Geometry check sheet. Reference: the model listing, model coordinates, mm. A direction names the side the tool comes from. Coordinates: 2 decimals unless noted, no trailing zeros. Write each loop counter-clockwise with the first axis right and the second up, starting at its lowest first coordinate (ties: lowest second). Pieces come first, ordered by that corner, then holes. Notation, with made-up numbers: M 42,21 L 47,21 A25 cw 47,60 Z; hole C 50.25,19 d9. An arc over 180 degrees is marked long. Write each question's results on one line, items separated by ' | '.
```python
from build123d import *

# Parameters (mm, degrees)
SKETCH_1_W          = 15.8
SKETCH_1_H          = 15.600000042
EXTRUDE_2_DEPTH     = 6.4
CUT_EXTRUDE_1_DEPTH = 3.2
SKETCH_3_R          = 2.400000003
EXTRUDE_3_DEPTH     = 1.7
SKETCH_4_R          = 2.4
EXTRUDE_4_DEPTH     = 1.7
CUT_EXTRUDE_2_DEPTH = 1.8
SKETCH_6_R          = 2.5
CUT_EXTRUDE_3_DEPTH = 1.8


with BuildPart() as part:
    # Эскиз1 → Бобышка-Вытянуть2 (new body)
    with BuildSketch(Plane(origin=(0, 0, 0), x_dir=(1, 0, 0), z_dir=(0, 1, 0))):
        Rectangle(SKETCH_1_W, SKETCH_1_H)
    extrude(amount=EXTRUDE_2_DEPTH)

    # Эскиз2 → Вырез-Вытянуть1 (cut)
    with BuildSketch(Plane(origin=(0, 6.4, 0), x_dir=(1, 0, 0), z_dir=(0, 1, 0))):
        Polygon((7.9, 0), (0, 0), (-7.9, 0), (-7.9, -7.800000021), (7.9, -7.800000021), align=None)
    extrude(amount=-CUT_EXTRUDE_1_DEPTH, mode=Mode.SUBTRACT)

    # Эскиз3 → Бобышка-Вытянуть3 (add)
    with BuildSketch(Plane(origin=(0, 3.2, 0), x_dir=(1, 0, 0), z_dir=(0, 1, 0))):
        with Locations(Location((-4, -3.900000021, 0), (0, 0, 270))):
            Circle(SKETCH_3_R)
        with Locations(Location((3.874, -3.900000021, 0), (0, 0, 270))):
            Circle(SKETCH_3_R)
    extrude(amount=EXTRUDE_3_DEPTH)

    # Эскиз4 → Бобышка-Вытянуть4 (add)
    with BuildSketch(Plane(origin=(0, 6.4, 0), x_dir=(1, 0, 0), z_dir=(0, 1, 0))):
        with Locations(Location((-4, 3.900000021, 0), (0, 0, 270))):
            Circle(SKETCH_4_R)
        with Locations(Location((3.874, 3.900000021, 0), (0, 0, 270))):
            Circle(SKETCH_4_R)
    extrude(amount=EXTRUDE_4_DEPTH)

    # Эскиз5 → Вырез-Вытянуть2 (cut)
    with BuildSketch(Plane.XZ):
        with BuildLine():
            ThreePointArc((2.241714395, 5.006669145), (0, 6.400000011), (-2.241714395, 5.006669145))
            Line((-2.241714395, 5.006669145), (0, 3.900000011))
            Line((0, 3.900000011), (2.241714395, 5.006669145))
        make_face()
        with BuildLine():
            Line((0, 3.900000011), (-2.241714395, 5.006669145))
            ThreePointArc((-2.241714395, 5.006669145), (-2.5, 3.900000011), (-2.241714395, 2.793330876))
            Line((-2.241714395, 2.793330876), (0, 3.900000011))
        make_face()
        with BuildLine():
            Line((0, 3.900000011), (-2.241714395, 2.793330876))
            ThreePointArc((-2.241714395, 2.793330876), (0, 1.400000011), (2.241714395, 2.793330876))
            Line((2.241714395, 2.793330876), (0, 3.900000011))
        make_face()
        with BuildLine():
            Line((2.241714395, 5.006669145), (0, 3.900000011))
            Line((0, 3.900000011), (2.241714395, 2.793330876))
            ThreePointArc((2.241714395, 2.793330876), (2.434572446, 3.331794936), (2.5, 3.900000011))
            ThreePointArc((2.5, 3.900000011), (2.434572446, 4.468205085), (2.241714395, 5.006669145))
        make_face()
    extrude(amount=-CUT_EXTRUDE_2_DEPTH, mode=Mode.SUBTRACT)

    # Эскиз6 → Вырез-Вытянуть3 (cut)
    with BuildSketch(Plane.XZ):
        with Locations(Location((0, -3.934549789, 0), (0, 0, 270))):
            Circle(SKETCH_6_R)
    extrude(amount=-CUT_EXTRUDE_3_DEPTH, mode=Mode.SUBTRACT)


solid = part.part
```
Q1. Sectioned sample at C-C on z = -3.75. Record the cut outline in (x, y).
Geometry check:
outline: M -7.9,0 L -2.49,0 L -2.49,1.8 L 2.49,1.8 L 2.49,0 L 7.9,0 L 7.9,6.4 L 6.27,6.4 L 6.27,8.1 L 1.48,8.1 L 1.48,6.4 L -1.6,6.4 L -1.6,8.1 L -6.4,8.1 L -6.4,6.4 L -7.9,6.4 Z
Q2. Mould release check, pull along X, two halves, no side actions. Record for faces 1 (the flat face through (-7.9, 2, -2)), 2 (the flat face through (0, 3, -7.8)), 3 (the flat face through (0, 3.2, 4)): pulls with the +X half, pulls with the -X half, needs draft (parallel to the pull), parting line crosses it, or undercut.
Geometry check:
face 1: pulls with the -X half | face 2: needs draft | face 3: undercut
Q3. Sectioned sample at B-B on x = 0. Record the cut outline in (y, z), and give its area (3 significant figures).
Geometry check:
outline: M 0,-7.8 L 6.4,-7.8 L 6.4,0 L 3.2,0 L 3.2,7.8 L 0,7.8 L 0,6.4 L 1.8,6.4 L 1.8,1.4 L 0,1.4 L 0,-1.43 L 1.8,-1.43 L 1.8,-6.43 L 0,-6.43 Z | area: 56.9 mm2
Q4. Access from +Z, -Z, +X, -X, +Y, -Y to the whole of each face (thin tool, end or side, straight path). Record for faces 4 (the flat face through (0, 6.4, -4)), 5 (the flat face through (-4, 4.9, 4)), 6 (the flat face through (0, 1.8, -4)), 7 (the flat face through (0, 5, 0)).
Geometry check:
face 4: +Y | face 5: +Z, +X, -X, +Y | face 6: -Y | face 7: +X, -X, +Y
Q5. Depth check by flat-ended pin: P1, Ø4, axis at x = -2.5, z = 4, coming from the +Y side; P2, Ø2.5, axis at x = 0, z = -4, coming from the -Y side; P3, Ø1.5, axis at x = 5, z = 0.5, coming from the +Y side. Enter the tip coordinate at first touch or a pass-through.
Geometry check:
P1: stops at y = 4.9 | P2: stops at y = 1.8 | P3: stops at y = 6.4
Q6. Scan lines: probe 1 along Z at (x, y) = (0.25, 1.5); probe 2 along Y at (x, z) = (-1.75, 7); probe 3 along Y at (x, z) = (-1.75, -1.75). Record each from-to range of solid material in increasing order.
Geometry check:
probe 1: z = -7.8 to -6.42, -1.45 to 1.41, 6.39 to 7.8 | probe 2: y = 0 to 3.2 | probe 3: y = 0 to 6.4
Q7. Sectioned sample at A-A on y = 1.25. Record the cut outline in (x, z), and give its area (3 significant figures).
Geometry check:
outline: M -7.9,-7.8 L 7.9,-7.8 L 7.9,7.8 L -7.9,7.8 Z; hole C 0,-3.93 d5; hole C 0,3.9 d5 | area: 207 mm2
Q8. Sectioned sample at D-D on y = 4.5. Record the cut outline in (x, z), and give its area (3 significant figures).
Geometry check:
outline: M -7.9,-7.8 L 7.9,-7.8 L 7.9,0 L -7.9,0 Z; C -4,3.9 d4.8; C 3.87,3.9 d4.8 | area: 159 mm2
